from build123d import *

# Parameters (mm, degrees)
EXTRUDE_1_DEPTH     = 145
SKETCH_2_R          = 3
CUT_EXTRUDE_1_DEPTH = 11
EXTRUDE_2_DEPTH     = 23
SKETCH_4_W          = 60
SKETCH_4_H          = 40
EXTRUDE_3_DEPTH     = 1.5
SKETCH_5_R          = 1.65
CUT_EXTRUDE_2_DEPTH = 12.5
CUT_EXTRUDE_3_DEPTH = 7
SKETCH_8_W          = 35
SKETCH_8_H          = 6
CUT_EXTRUDE_5_DEPTH = 12.5
CUT_EXTRUDE_6_DEPTH = 11


with BuildPart() as part:
    # 草图1 → 凸台-拉伸1 (new body)
    with BuildSketch(Plane(origin=(0, 0, 0), x_dir=(0, 0, -1), z_dir=(1, 0, 0))):
        with BuildLine():
            Line((-20, 10), (-20, 0))
            Line((-20, 0), (20, 0))
            Line((20, 0), (20, 10))
            Line((20, 10), (11.489125293, 10))
            ThreePointArc((11.489125293, 10), (0, 6), (-11.489125293, 10))
            Line((-11.489125293, 10), (-20, 10))
        make_face()
    extrude(amount=EXTRUDE_1_DEPTH)

    # 草图2 → 切除-拉伸1 (cut, through all)
    with BuildSketch(Plane.XZ):
        with Locations((137.5, -15)):
            Circle(SKETCH_2_R)
        with Locations((113.5, -15)):
            Circle(SKETCH_2_R)
        with Locations((113.5, 15)):
            Circle(SKETCH_2_R)
        with Locations((137.5, 15)):
            Circle(SKETCH_2_R)
        with Locations((7.5, 15)):
            Circle(SKETCH_2_R)
        with Locations((31.5, 15)):
            Circle(SKETCH_2_R)
        with Locations((31.5, -15)):
            Circle(SKETCH_2_R)
        with Locations((7.5, -15)):
            Circle(SKETCH_2_R)
    extrude(amount=-CUT_EXTRUDE_1_DEPTH, mode=Mode.SUBTRACT)

    # 草图3 → 凸台-拉伸2 (add)
    with BuildSketch(Plane(origin=(27, 0, 0), x_dir=(0, 0, -1), z_dir=(1, 0, 0))):
        with BuildLine():
            Line((11.489125293, 10), (7.874007874, 10))
            ThreePointArc((7.874007874, 10), (0, 8), (-7.874007874, 10))
            Line((-7.874007874, 10), (-11.489125293, 10))
            ThreePointArc((-11.489125293, 10), (0, 6), (11.489125293, 10))
        make_face()
    extrude_2 = extrude(amount=EXTRUDE_2_DEPTH)

    # 镜向1: 凸台-拉伸2 across plane
    add(extrude_2.mirror(Plane(origin=(72.5, 0, 0), x_dir=(0, 0, 1), z_dir=(1, 0, 0))))

    # 草图4 → 凸台-拉伸3 (add)
    with BuildSketch(Plane.XZ):
        with Locations((72.5, 0)):
            Rectangle(SKETCH_4_W, SKETCH_4_H)
    extrude(amount=EXTRUDE_3_DEPTH)

    # 草图5 → 切除-拉伸2 (cut, through all)
    with BuildSketch(Plane.XZ.offset(1.5)):
        with Locations((57.5, 10)):
            Circle(SKETCH_5_R)
        with Locations((57.5, -10)):
            Circle(SKETCH_5_R)
        with Locations((87.5, -10)):
            Circle(SKETCH_5_R)
        with Locations((87.5, 10)):
            Circle(SKETCH_5_R)
    extrude(amount=-CUT_EXTRUDE_2_DEPTH, mode=Mode.SUBTRACT)

    # 草图6 → 切除-拉伸3 (cut)
    with BuildSketch(Plane(origin=(0, 10, 0), x_dir=(1, 0, 0), z_dir=(0, 1, 0))):
        Polygon((60.559956427, 10), (59.029978213, 12.65), (55.970021787, 12.65), (54.440043573, 10), (55.970021787, 7.35), (59.029978213, 7.35), align=None)
        Polygon((90.559956427, 10), (89.029978213, 12.65), (85.970021787, 12.65), (84.440043573, 10), (85.970021787, 7.35), (89.029978213, 7.35), align=None)
        Polygon((60.559956427, -10), (59.029978213, -7.35), (55.970021787, -7.35), (54.440043573, -10), (55.970021787, -12.65), (59.029978213, -12.65), align=None)
        Polygon((90.559956427, -10), (89.029978213, -7.35), (85.970021787, -7.35), (84.440043573, -10), (85.970021787, -12.65), (89.029978213, -12.65), align=None)
    extrude(amount=-CUT_EXTRUDE_3_DEPTH, mode=Mode.SUBTRACT)

    # 草图8 → 切除-拉伸5 (cut, through all)
    with BuildSketch(Plane(origin=(0, 10, 0), x_dir=(1, 0, 0), z_dir=(0, 1, 0))):
        with Locations((72.5, -17)):
            Rectangle(SKETCH_8_W, SKETCH_8_H)
    extrude(amount=-CUT_EXTRUDE_5_DEPTH, mode=Mode.SUBTRACT)

    # 草图9 → 切除-拉伸6 (cut, through all)
    with BuildSketch(Plane.XZ):
        with BuildLine():
            Line((133.75, -2.5), (126.25, -2.5))
            Line((126.25, -2.5), (126.25, -10))
            ThreePointArc((126.25, -10), (123.75, -12.5), (121.25, -10))
            Line((121.25, -10), (121.25, -2.5))
            Line((121.25, -2.5), (113.75, -2.5))
            ThreePointArc((113.75, -2.5), (111.25, 0), (113.75, 2.5))
            Line((113.75, 2.5), (121.25, 2.5))
            Line((121.25, 2.5), (121.25, 10))
            ThreePointArc((121.25, 10), (123.75, 12.5), (126.25, 10))
            Line((126.25, 10), (126.25, 2.5))
            Line((126.25, 2.5), (133.75, 2.5))
            ThreePointArc((133.75, 2.5), (136.25, 0), (133.75, -2.5))
        make_face()
        with BuildLine():
            Line((23.75, -2.5), (23.75, -10))
            ThreePointArc((23.75, -10), (21.25, -12.5), (18.75, -10))
            Line((18.75, -10), (18.75, -2.5))
            Line((18.75, -2.5), (11.25, -2.5))
            ThreePointArc((11.25, -2.5), (8.75, 0), (11.25, 2.5))
            Line((11.25, 2.5), (18.75, 2.5))
            Line((18.75, 2.5), (18.75, 10))
            ThreePointArc((18.75, 10), (21.25, 12.5), (23.75, 10))
            Line((23.75, 10), (23.75, 2.5))
            Line((23.75, 2.5), (31.25, 2.5))
            ThreePointArc((31.25, 2.5), (33.75, 0), (31.25, -2.5))
            Line((31.25, -2.5), (23.75, -2.5))
        make_face()
    extrude(amount=-CUT_EXTRUDE_6_DEPTH, mode=Mode.SUBTRACT)


solid = part.part
The model under review builds one solid part; all positions refer to its coordinate system, in mm. A direction names the side the tool comes from. Give positions to 0.01 mm unless a question says otherwise; leave off trailing zeros. Write each loop counter-clockwise with the first axis right and the second up, starting at its lowest first coordinate (ties: lowest second). Pieces come first, ordered by that corner, then holes.
1. Tool access review of faces 4 (the flat face through (89, 3, -11)), 5 (the cylindrical face through (137, 6, 0)), 6 (the flat face through (23.75, 3, -6)): name each direction out of +Z, -Z, +X, -X, +Y, -Y from which nothing blocks a thin tool from reaching the whole face with its end or side.
2. Add section A-A, the plane x = 7.5. Write out the cut boundary in (y, z).
3. Add section C-C, the plane x = 65. Write out the cut boundary in (y, z), plus the area to 3 significant figures.
4. Add section D-D, the plane y = 1.25. Count the separate pieces of the cut face and the enclosed holes in it, plus the area to 3 significant figures.
5. Wall thickness on L1, parallel to Z at x = 89, y = 5.5; L2, parallel to X at y = 5.25, z = -4; L3, parallel to Z at x = 87.5, y = 1.2: over which ranges is each line inside the solid? List them lowest first.
6. Add section B-B, the plane z = 0. Write out the cut boundary in (x, y), plus the area to 3 significant figures.
7. Draft analysis for pull direction Z (two halves, no side actions). For faces 1 (the flat face through (121.25, 3, 6)), 2 (the flat face through (27, 4, 20)), 3 (the flat face through (71, 10, -15)), state which applies: +Z half, -Z half, draft (parallel to the pull), parting line (faces both ways), or undercut.
8. For P1, Ø7, axis at x = 113.5, z = 15, coming from the +Y side; P2, Ø8, axis at x = 113.5, z = -15, coming from the -Y side; P3, Ø3.5, axis at x = 88, y = 6, coming from the +Z side; P4, Ø1.1, axis at y = 9, z = -5.5, coming from the -X side, all flat-tipped, find the tip position at first contact; note any pin that passes through.
Worked answers:
1. face 4: +Y
1. face 5: +X, +Y
1. face 6: +Y, -Y
2. outline: (0, -20) - (10, -20) - (10, -18) - (0, -18) - close; (0, -12) - (10, -12) - (10, -11.49) arc R18.5 cw to (10, 11.49) - (10, 12) - (0, 12) - close; (0, 18) - (10, 18) - (10, 20) - (0, 20) - close
3. outline: (-1.5, -20) - (10, -20) - (10, -11.49) arc R18.5 cw to (10, 11.49) - (10, 14) - (-1.5, 14) - close
3. area: 328 mm2
4. separate pieces: 1
4. enclosed holes: 14
4. area: 4,900 mm2
5. L1: z = -20 to -12.65, -7.35 to 7.35, 12.65 to 14
5. L2: x = 0 to 18.75, 23.75 to 121.25, 126.25 to 145
5. L3: z = -20 to -11.65, -8.35 to 8.35, 11.65 to 14
6. outline: (0, 0) - (8.75, 0) - (8.75, 6) - (0, 6) - close; (33.75, 0) - (42.5, 0) - (42.5, -1.5) - (102.5, -1.5) - (102.5, 0) - (111.25, 0) - (111.25, 8) - (95, 8) - (95, 6) - (50, 6) - (50, 8) - (33.75, 8) - close; (136.25, 0) - (145, 0) - (145, 6) - (136.25, 6) - close
6. area: 725 mm2
7. face 1: undercut
7. face 2: +Z half
7. face 3: draft
8. P1: stops at y = 10
8. P2: stops at y = 0
8. P3: stops at z = 14
8. P4: stops at x = 27
